Geometry: see drawing. Coordinates: mm, zero at the bounding-box minimum. A direction names the side the tool comes from. Give positions to 0.01 mm unless a question says otherwise; leave off trailing zeros. Loops run counter-clockwise (first coordinate to the right, second up) from the corner with the lowest first, then second, coordinate; pieces in that order, holes last. Notation, with made-up numbers: (29, 68.25) -> (53, 68.25) arc R18 ccw to (53, 95.25) -> close; hole circle Ø2 at (-32, 57.25). An arc over 180 degrees is marked (long way). Return JSON: item names as keys, results as strings. Group by question number.
(1) Cut plane D-D on y = 3.25. Return loops of the section in (x, z).
(2) Draft query along X for the marked faces 4, 5 and 6. Return one class per face: released by +X, released by -X, zero draft, split by the parting line, or undercut.
(3) Cut plane A-A on x = 9.5. Return loops of the section in (y, z).
(4) Access query for the marked faces 1, 2 and 3. Directions: +Z, -Z, +X, -X, +Y, -Y. A direction counts if a zero-diameter tool reaches every point of the face in a straight line with its end or side. Return the directions, or none.
(5) Cut plane C-C on z = 9.5. Return loops of the section in (x, y).
(6) Cut plane B-B on y = 1.25. Return loops of the section in (x, z).
(7) Pin query (flat end, axial travel): pin 1 (4 mm diameter, centred on x = 8, y = 5.5, fed in from -Z); pin 2 (2 mm diameter, centred on x = 5.5, y = 7, fed in from -Z) (1 decimal); pin 3 (2.5 mm diameter, centred on x = 12, y = 4.5, fed in from +Z) (1 decimal); pin 4 (3.5 mm diameter, centred on x = 9, z = 10, fed in from +Y). Return the tip coordinate at first contact, or that it passes through.
(8) Ray query, line 1 (Z direction, x = 9.5, y = 1.5); line 2 (Y direction, x = 6.5, z = 7.5); line 3 (Z direction, x = 9.5, y = 7.05) (1 decimal). Return the intervals inside material, ascending. Write a range as from..to.
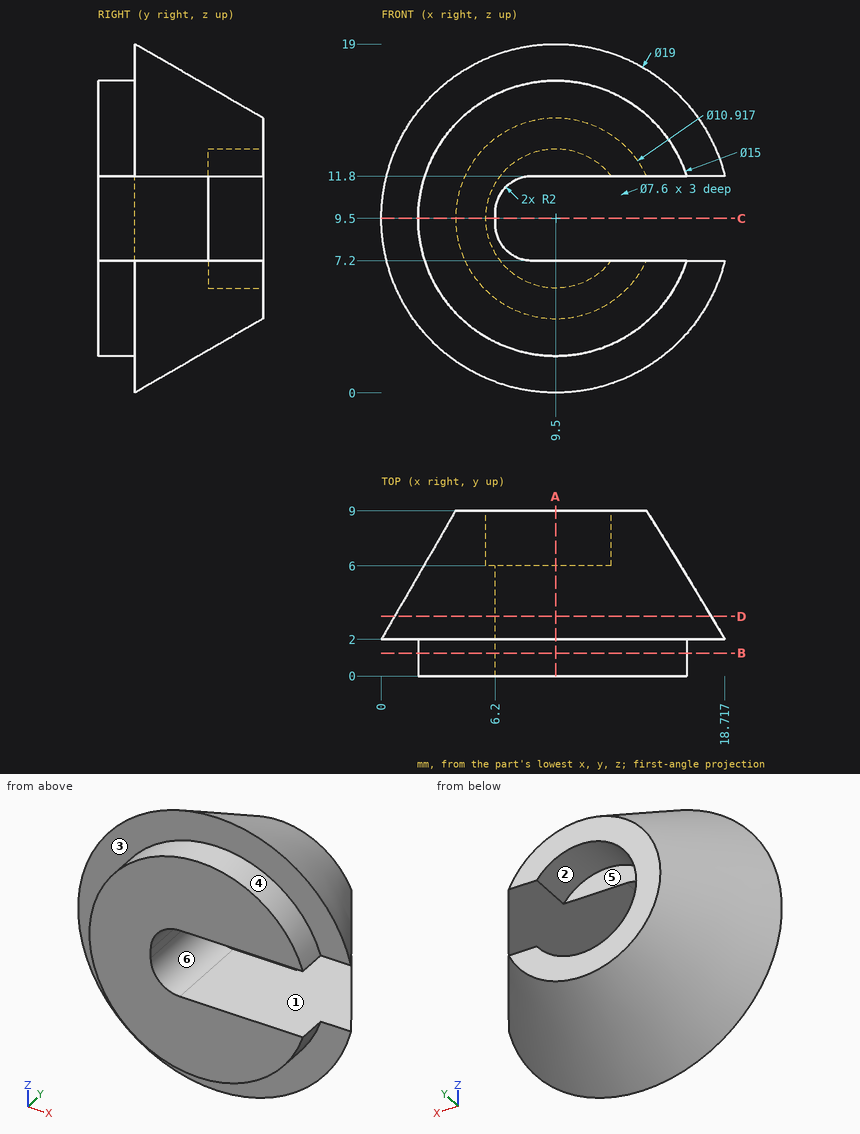
Answers:
{
 "1": {"outline": "(6.2, 9.2) -> (6.2, 9.8) arc R2 cw to (8.2, 11.8) -> (17.97, 11.8) arc R8.78 ccw (long way) to (17.97, 7.2) -> (8.2, 7.2) arc R2 cw to start"},
 "2": {"face 4": "split by the parting line", "face 5": "undercut", "face 6": "released by +X"},
 "3": {"outline": "(0, 2) -> (2, 2) -> (2, 0) -> (9, 4.04) -> (9, 5.7) -> (6, 5.7) -> (6, 7.2) -> (0, 7.2) -> close; (0, 11.8) -> (6, 11.8) -> (6, 13.3) -> (9, 13.3) -> (9, 14.96) -> (2, 19) -> (2, 17) -> (0, 17) -> close"},
 "4": {"face 1": "+X, +Y, -Y", "face 2": "+Y", "face 3": "-Y"},
 "5": {"outline": "(0, 2) -> (2, 2) -> (2, 0) -> (6.2, 0) -> (6.2, 6) -> (5.7, 6) -> (5.7, 9) -> (4.04, 9) -> close"},
 "6": {"outline": "(6.2, 9.2) -> (6.2, 9.8) arc R2 cw to (8.2, 11.8) -> (16.64, 11.8) arc R7.5 ccw (long way) to (16.64, 7.2) -> (8.2, 7.2) arc R2 cw to start"},
 "7": {"pin 1": "z = 0.96", "pin 2": "z = 3.3", "pin 3": "z = 18", "pin 4": "through"},
 "8": {"line 1": "2..7.2, 11.8..17", "line 2": "0..6", "line 3": "2.9..5.7, 13.3..16.1"}
}
